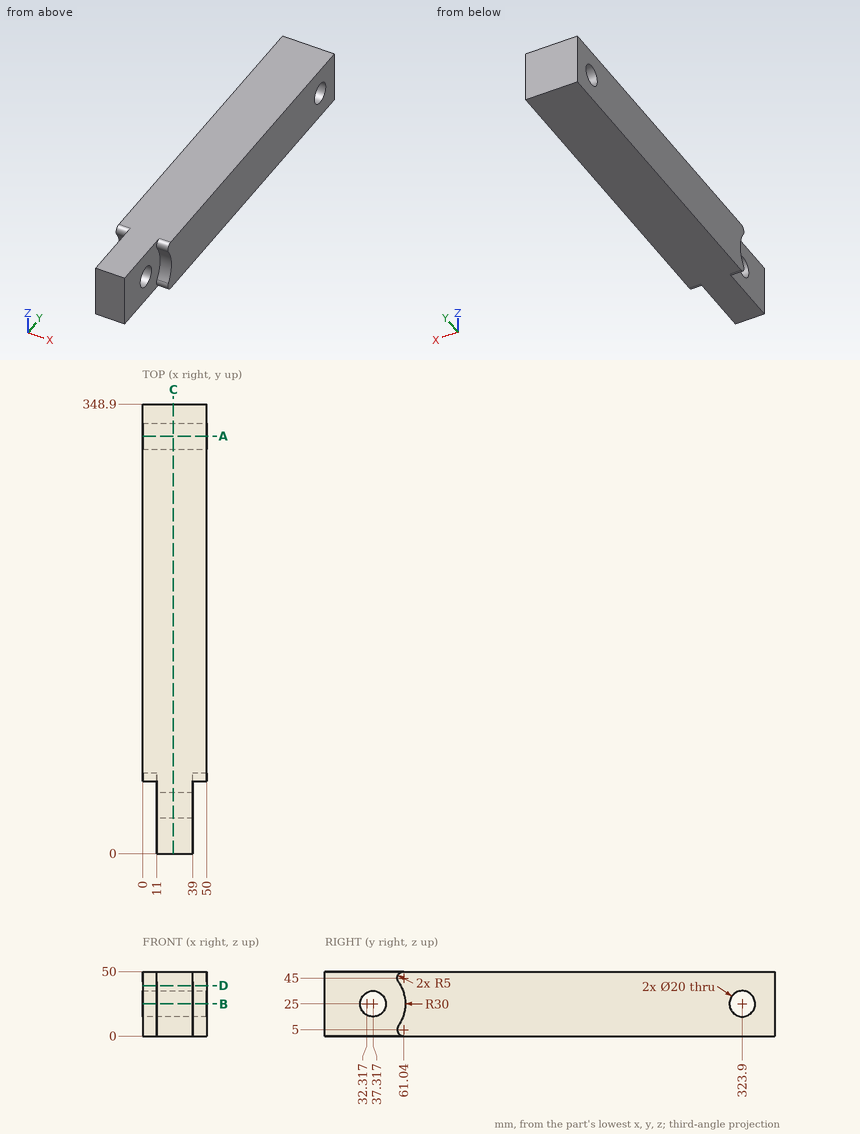
Print and shaded views of the part. All mm, measured from the part's lowest x, y and z. Coordinates: 2 decimals unless noted, no trailing zeros. Order: outer loops, then holes, each group sorted by start corner. A loop starts at its lowest first (then second) coordinate and runs counter-clockwise, first axis right, second up.
Item 1: Saw through at B-B on z = 25. List the corners of the cut face in (x, y).
Filled in:
outline: (0, 62.32) - (11, 62.32) - (11, 47.32) - (39, 47.32) - (39, 62.32) - (50, 62.32) - (50, 313.9) - (0, 313.9) - close; (0, 333.9) - (50, 333.9) - (50, 348.9) - (0, 348.9) - close; (11, 0) - (39, 0) - (39, 27.32) - (11, 27.32) - close
Item 2: Saw through at A-A on y = 323.9. List the corners of the cut face in (x, z), then the cut area to 3 significant figures.
Filled in:
outline: (0, 0) - (50, 0) - (50, 15) - (0, 15) - close; (0, 35) - (50, 35) - (50, 50) - (0, 50) - close
area: 1,500 mm2
Item 3: Saw through at D-D on z = 39. List the corners of the cut face in (x, y), then the cut area to 4 significant figures.
Filled in:
outline: (0, 58.85) - (11, 58.85) - (11, 0) - (39, 0) - (39, 58.85) - (50, 58.85) - (50, 348.9) - (0, 348.9) - close
area: 16,150 mm2
Item 4: Saw through at C-C on x = 24. List the corners of the cut face in (y, z).
Filled in:
outline: (0, 0) - (348.9, 0) - (348.9, 50) - (0, 50) - close; hole circle Ø20 at (37.32, 25); hole circle Ø20 at (323.9, 25)
Item 5: Drop flat-ended pins along their axis: pin 1 Ø15 at (y, z) = (29.5, 28.5) entering from +X; pin 2 Ø15 at (y, z) = (31.5, 19.5) entering from -X. Give the stop position or say it passes through.
Filled in:
pin 1: stops at x = 39
pin 2: stops at x = 11
Item 6: Drill centre lines: L1, parallel to Y at x = 14, z = 25; L2, parallel to Y at x = 38, z = 18.5 (1 decimal); L3, parallel to Z at x = 34, y = 323. Where is each one in solid material? Low to high.
Filled in:
L1: y = 0 to 27.32, 47.32 to 313.9, 333.9 to 348.9
L2: y = 0 to 29.7, 44.9 to 316.3, 331.5 to 348.9
L3: z = 0 to 15.04, 34.96 to 50
